Could you check a few things on this drawing? It's one solid part, dimensions in mm from its lowest x, y, z. A direction names the side the tool comes from. Round coordinates to 2 decimals unless told otherwise and drop trailing zeros. Write each loop counter-clockwise with the first axis right and the second up, starting at its lowest first coordinate (ties: lowest second). Pieces come first, ordered by that corner, then holes. Notation, with made-up numbers: (-23, -27.5) - (15, -27.5) arc R29 ccw to (15, 9.5) - close; hole circle Ø10 at (-22.75, 14.25). An arc over 180 degrees is marked (long way). Write item = value, one per line. Start each with the question number.
Item 1: If we section it at C-C (z = 7): Please give me the cut outline in (x, y).
Item 2: If we section it at B-B (x = 10.5): Please give me the cut outline in (y, z).
Item 3: For P1, Ø2, axis at y = 5.5, z = 16, coming from the -X side; P2, Ø3, axis at x = 6, z = 17.5, coming from the -Y side; P3, Ø2, axis at y = 4.5, z = 8, coming from the -X side, each with a flat end and sliding along its axis, tell me the tip position at first contact or that it passes through.
Item 4: Thinking about a two-plate mould opening in X: for the marked faces 3, 4 and 5, which applies, pulls with the +X half, pulls with the -X half, needs draft (parallel to the pull), parting line crosses it, or undercut?
Item 5: If we section it at D-D (y = 1.5): Please give me the cut outline in (x, z), and give its area (3 significant figures).
Item 6: If I drill on line 1 along Z through (x, y) = (10.5, 1.85); line 2 along X through (y, z) = (6, 10.5), over which ranges is the centre line in solid material (lowest first)? Write a range as [from, to].
Item 7: Which directions (+Z, -Z, +X, -X, +Y, -Y) give clear straight access to the entire face, cutting with the end or side of a thin tool? Please do the marked faces 1 and 2.
Item 8: If we section it at A-A (z = 10.5): Please give me the cut outline in (x, y), and give its area (3 significant figures).
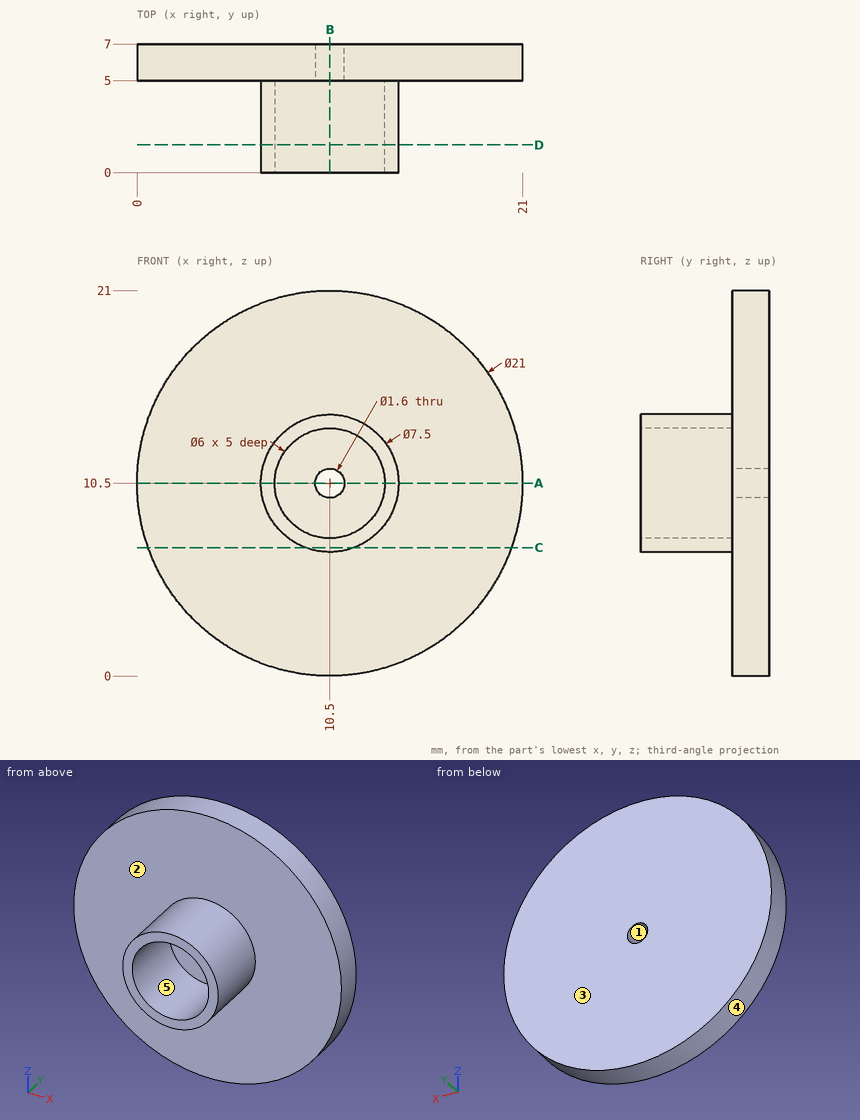
Reply:
q1.outline = (0.6, 5) - (9.15, 5) - (9.15, 0) - (11.85, 0) - (11.85, 5) - (20.4, 5) - (20.4, 7) - (0.6, 7) - close
q2.outline = (0, 6.75) - (5, 6.75) - (5, 0) - (7, 0) - (7, 9.7) - (5, 9.7) - (5, 7.5) - (0, 7.5) - close; (0, 13.5) - (5, 13.5) - (5, 11.3) - (7, 11.3) - (7, 21) - (5, 21) - (5, 14.25) - (0, 14.25) - close
q3.P1 = 1.01
q3.P2 = 5
q3.P3 = 0.13
q4.face_3 = needs draft
q4.face_4 = parting line crosses it
q4.face_5 = undercut
q5.outline = circle Ø7.5 at (10.5, 10.5); hole circle Ø6 at (10.5, 10.5)
q5.area = 15.9 mm2
q6.line_1 = [6.75, 7.5], [13.5, 14.25]
q6.line_2 = [0, 9.7], [11.3, 21]
q7.face_1 = +Y, -Y
q7.face_2 = -Y
q8.outline = (0, 5) - (6.75, 5) - (6.75, 0) - (7.5, 0) - (7.5, 5) - (9.7, 5) - (9.7, 7) - (0, 7) - close; (11.3, 5) - (13.5, 5) - (13.5, 0) - (14.25, 0) - (14.25, 5) - (21, 5) - (21, 7) - (11.3, 7) - close
q8.area = 46.3 mm2
